Design review of the part built by this model. Coordinates are the model's own, in mm. Face numbers are marked on the shaded views. A direction names the side the tool comes from. Round coordinates to 2 decimals unless told otherwise and drop trailing zeros. Loops run counter-clockwise (first coordinate to the right, second up) from the corner with the lowest first, then second, coordinate; pieces in that order, holes last. Notation, with made-up numbers: M -3.75,59 L 27.25,59 A20 cw 27.25,73 Z; hole C 63.25,46 d8. An arc over 180 degrees is marked long. Use a Markdown table: item, result.
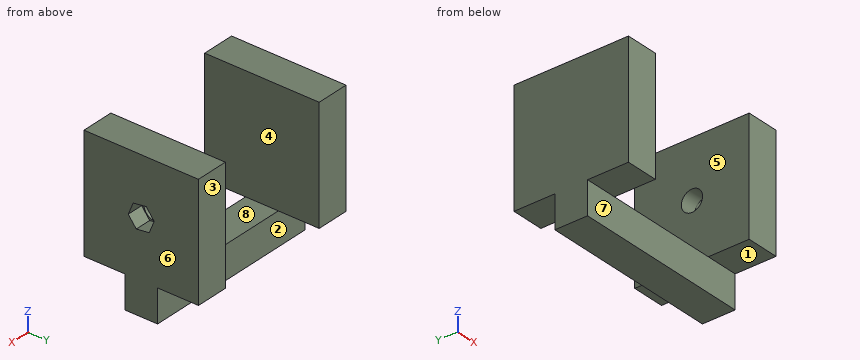
from build123d import *

# Parameters (mm, degrees)
F1_DEPTH  = 10
F2_W      = 12.5
F2_H      = 35
F3_DEPTH  = 10
F4_W      = 12.5
F4_H      = 35
F5_DEPTH  = 10
F6_R      = 3.25
F7_DEPTH  = 10
F9_R      = 3.25
F10_DEPTH = 5


with BuildPart() as f1:
    # F0 (on Front) → F1 (new body)
    with BuildSketch(Plane.XZ):
        Polygon((-12.7756818049, 38.8276573637), (-22.7756818049, 38.8276573637), (-22.7756818049, -6.1723426363), (32.2243181951, -6.1723426363), (32.2243181951, 38.8276573637), (22.2243181951, 38.8276573637), (22.2243181951, 3.8276573637), (-12.7756818049, 3.8276573637), align=None)
    extrude(amount=F1_DEPTH)

    # F2 (on face) → F3 (join)
    with BuildSketch(Plane.YZ.offset(32.2243181951)):
        with Locations((-16.25, 21.3276573637)):
            Rectangle(F2_W, F2_H)
        with Locations((6.25, 21.3276573637)):
            Rectangle(F2_W, F2_H)
    extrude(amount=-F3_DEPTH)

    # F4 (on face) → F5 (join)
    with BuildSketch(Plane(origin=(-22.7756818049, 0, 0), x_dir=(0, -1, 0), z_dir=(-1, 0, 0))):
        with Locations((-6.25, 21.3276573637)):
            Rectangle(F4_W, F4_H)
        with Locations((16.25, 21.3276573637)):
            Rectangle(F4_W, F4_H)
    extrude(amount=-F5_DEPTH)

    # F6 (on face) → F7 (cut)
    with BuildSketch(Plane.YZ.offset(32.2243181951)):
        with Locations((-5, 21.3276573637)):
            Circle(F6_R)
    extrude(amount=-F7_DEPTH, mode=Mode.SUBTRACT)

    # F9 (on face) → F10 (cut)
    with BuildSketch(Plane.YZ.offset(32.2243181951)):
        Polygon((-1.0361268053, 21.8640427628), (-3.4825867845, 25.0286649472), (-7.4464599792, 24.4922795481), (-8.9638731947, 20.7912719646), (-6.5174132155, 17.6266497802), (-2.5535400208, 18.1630351792), align=None)
        with Locations((-5, 21.3276573637)):
            Circle(F9_R, mode=Mode.SUBTRACT)
    extrude(amount=-F10_DEPTH, mode=Mode.SUBTRACT)


solid = f1.part
1. Take a section at A-A on z = 16.5. Give the boundary of the cut face in (x, y).
Check values:
| item | result |
|---|---|
| outline | M -22.78,-22.5 L -12.78,-22.5 L -12.78,12.5 L -22.78,12.5 Z; M 22.22,-22.5 L 32.22,-22.5 L 32.22,12.5 L 22.22,12.5 Z |
2. Wall thickness on line 1 along Z through (x, y) = (24.5, -5); line 2 along X through (y, z) = (-16, 4); line 3 along Z through (x, y) = (23.5, 8): over which ranges is each line inside the solid? List them lowest first. Write a range as from..to.
Check values:
| item | result |
|---|---|
| line 1 | z = -6.17..18.08, 24.58..38.83 |
| line 2 | x = -22.78..-12.78, 22.22..32.22 |
| line 3 | z = 3.83..38.83 |
3. The part is to be moulded in two halves that separate along X. For the marked faces 5, 6, 7 and 8, say which applies: pulls with the +X half, pulls with the -X half, needs draft (parallel to the pull), parting line crosses it, or undercut.
Check values:
| item | result |
|---|---|
| face 5 | undercut |
| face 6 | pulls with the +X half |
| face 7 | needs draft |
| face 8 | undercut |
4. Take a section at B-B on y = 10. Give the boundary of the cut face in (x, z).
Check values:
| item | result |
|---|---|
| outline | M -22.78,3.83 L -12.78,3.83 L -12.78,38.83 L -22.78,38.83 Z; M 22.22,3.83 L 32.22,3.83 L 32.22,38.83 L 22.22,38.83 Z |
5. Take a section at C-C on x = -15. Give the boundary of the cut face in (y, z), and give its area (4 significant figures).
Check values:
| item | result |
|---|---|
| outline | M -22.5,3.83 L -10,3.83 L -10,-6.17 L 0,-6.17 L 0,3.83 L 12.5,3.83 L 12.5,38.83 L -22.5,38.83 Z |
| area | 1,325 mm² |
6. Take a section at D-D on y = -5. Give the boundary of the cut face in (x, z), and give its area (3 significant figures).
Check values:
| item | result |
|---|---|
| outline | M -22.78,-6.17 L 32.22,-6.17 L 32.22,17.83 L 27.22,17.83 L 27.22,18.08 L 22.22,18.08 L 22.22,3.83 L -12.78,3.83 L -12.78,38.83 L -22.78,38.83 Z; M 22.22,24.58 L 27.22,24.58 L 27.22,24.82 L 32.22,24.82 L 32.22,38.83 L 22.22,38.83 Z |
| area | 1,180 mm² |
7. Insertion check: pin 1 (8 mm diameter, centred on x = 10, z = 0.5, fed in from +Y); pin 2 (3 mm diameter, centred on x = -6, z = 0.5, fed in from -Y); pin 3 (1.5 mm diameter, centred on x = 19, y = -11, fed in from +Z); pin 4 (3 mm diameter, centred on x = -1.5, y = -4.5, fed in from +Z). Each pin has a flat end and moves straight along its axis. Give the tip position at first contact, or say it passes through.
Check values:
| item | result |
|---|---|
| pin 1 | stops at y = 0 |
| pin 2 | stops at y = -10 |
| pin 3 | passes through |
| pin 4 | stops at z = 3.83 |
8. Machinability: for the marked faces 1, 2, 3 and 4, which of the approach directions +Z, -Z, +X, -X, +Y, -Y give a long, thin tool a straight path to every point of the face, cutting with its end or side? Answer none if there is none.
Check values:
| item | result |
|---|---|
| face 1 | -Z, +X, -X, -Y |
| face 2 | -Z, +X, -X, +Y |
| face 3 | +Z, -Z, +X, -X, +Y |
| face 4 | +Z, +Y, -Y |
